Verification items for the finished model (mm, model axes). A direction names the side the tool comes from. Coordinates: 2 decimals unless noted, no trailing zeros. Write each loop counter-clockwise with the first axis right and the second up, starting at its lowest first coordinate (ties: lowest second). Pieces come first, ordered by that corner, then holes. Notation, with made-up numbers: M 80,78 L 89,78 A24 ccw 89,93 Z; hole C 17,41 d10. An arc over 180 degrees is marked long. Answer in a Markdown table with one row per item.
Autodesk Inventor part; units mm, degrees
ref_plane "YZ Plane" through (0, 0, 0) normal (1, 0, 0) x (0, 1, 0)
ref_plane "XZ Plane" through (0, 0, 0) normal (0, 1, 0) x (-1, 0, 0)
ref_plane "XY Plane" through (0, 0, 0) normal (0, 0, 1) x (1, 0, 0)
sketch "Sketch1" plane through (0, 0, 0) normal (0, 0, 1) x (1, 0, 0)
  line L0 (0, 0) -> (6.223, 0)
  line L1 (0, 0) -> (6.223, 0) construction
  line L2 (6.223, 0) -> (6.223, 38.1)
  line L3 (0, 0) -> (0.762, 0)
  line L4 (0.762, 0) -> (0.762, 8.255)
  line L5 (0.762, 8.255) -> (6.223, 28.635729)
  line L6 (6.223, 28.635729) -> (6.223, 38.1)
  line L7 (0, 0) -> (12.7, 0)
  line L8 (0, -8.9154) -> (0, 53.4924)
  line L9 (6.223, 38.1) -> (12.20332, 44.08032)
  line L10 (6.223, 38.1) -> (14.68045, 38.1) construction
  line L11 (12.20332, 44.08032) -> (12.7, 0)
  line L12 (12.7, 0) -> (12.7, 44.577)
  line L13 (12.7, 44.577) -> (6.223, 38.1)
  line L14 (6.223, 38.1) -> (0, 38.1)
  line L15 (0, 8.255) -> (0.762, 8.255)
  line L16 (0, 8.255) -> (0, 38.1)
  line L17 (6.223, 28.635729) -> (0, 28.635729)
  line L18 (0, 28.635729) -> (8.60425, 28.635729)
  line L19 (8.60425, 28.635729) -> (0.762, 8.255)
  line L20 (8.60425, 28.635729) -> (8.60425, 40.48125)
  dimension "d0" = 6.223
  dimension "d1" = 0
  dimension "d2" = 38.1
  dimension "d3" = 90
  dimension "d4" = 0.762
  dimension "d5" = 8.255
  dimension "d6" = 165
  dimension "d7" = 12.7
  dimension "d18" = 45
  dimension "d58" = 8.60425
sketch "Sketch1 outline for Revolution1" plane through (0, 0, 0) normal (0, 0, 1) x (1, 0, 0)
  line L0 (8.60425, 40.48125) -> (8.60425, 28.635729)
  line L1 (8.60425, 28.635729) -> (0.762, 8.255)
  line L2 (0.762, 8.255) -> (0.762, 0)
  line L3 (0.762, 0) -> (12.7, 0)
  line L4 (12.7, 0) -> (12.7, 44.577)
  line L5 (12.7, 44.577) -> (8.60425, 40.48125)
revolve "Revolution1" add sketch "Sketch1 outline for Revolution1" angle 360 about axis through (0, -10, 0) along (0, 1, 0)
sketch "Sketch3" plane through (0, 0, 0) normal (0, -1, 0) x (1, 0, 0)
  point P0 (0, 0)
  point P1 (0, 0)
hole "Hole2" at (0, 0, 0) direction (0, 1, 0) diameter 5.3594 depth 6.35
sketch "Sketch4" plane through (0, 0, 0) normal (1, 0, 0) x (0, 1, 0)
  line L0 (0, 12.7) -> (0, -12.7)
  line L1 (0, 12.7) -> (0, 7.9248)
  line L2 (0, 7.9248) -> (12.7, 7.9248)
  line L3 (0, -12.7) -> (0, -7.9248)
  line L4 (0, -7.9248) -> (12.7, -7.9248)
  point P0 (0, 0)
  dimension "d28" = 4.7752
  dimension "d29" = 12.7
  dimension "d30" = 4.7752
  dimension "d31" = 12.7
  dimension "d32" = 90
hole "Hole3" at (0, 12.7, 7.9248) at (0, 12.7, -7.9248) direction (-1, 0, 0) diameter 4.4958 end through all
mirror "Mirror1" about plane through (0, 0, 0) normal (1, 0, 0) of "Hole3"
equation "\"d47\" = 55deg"
equation "\"Sketch5_Pitch\" = 0.90714"
properties part number "catch vertical seal-tighttol-thread"
1) Thickness scan on L1, parallel to Z at x = 0, y = 7.8; L2, parallel to X at y = 3.5, z = 0; L3, parallel to Z at x = -4.25, y = 12.5. Record the ranges inside material, lowest first. Write a range as [from, to].
Response values:
| item | result |
|---|---|
| L1 | z = [-12.7, -0.76], [0.76, 12.7] |
| L2 | x = [-12.7, -2.68], [2.68, 12.7] |
| L3 | z = [-11.97, -10.16], [-5.69, 5.69], [10.16, 11.97] |
2) Sectioned sample at D-D (y = 33). Record the cut outline in (x, z), then the cut area to 3 significant figures.
Response values:
| item | result |
|---|---|
| outline | C 0,0 d25.4; hole C 0,0 d17.21 |
| area | 274 mm² |
3) Release check for a two-part mould opening along X. For faces 4 (the face through (12.114, 22.601, -3.815)), 5 (the face through (-1.92, 40.74, 8.65)), 6 (the face through (0.16, 12.8, -5.68)) record: +X half, -X half, draft (parallel to the pull), parting line (faces both ways), or undercut.
Response values:
| item | result |
|---|---|
| face 4 | parting line |
| face 5 | undercut |
| face 6 | draft |
4) Depth check by flat-ended pin: pin 1 (6 mm diameter, centred on y = 12.7, z = 7.92, fed in from -X); pin 2 (12 mm diameter, centred on x = 3, z = 8.5, fed in from -Y); pin 3 (1 mm diameter, centred on y = 8, z = 1, fed in from +X); pin 4 (1 mm diameter, centred on x = 1, y = 6, fed in from +Z). Enter the tip coordinate at first touch or a pass-through.
Response values:
| item | result |
|---|---|
| pin 1 | stops at x = -11.71 |
| pin 2 | stops at y = 0 |
| pin 3 | stops at x = 12.69 |
| pin 4 | stops at z = 12.69 |
5) Tool access check on faces 1 (the face through (0, 0, -3)), 2 (the face through (-1.87, 34.48, -8.4)), 3 (the face through (-0.118, 3.219, 2.677)). Record the directions out of +Z, -Z, +X, -X, +Y, -Y that give a thin tool (end or side, any length) a straight path to the whole face; none if there is none.
Response values:
| item | result |
|---|---|
| face 1 | +Z, -Z, +X, -X, -Y |
| face 2 | +Y |
| face 3 | -Y |
6) Sectioned sample at C-C (y = 12.7). Record the cut outline in (x, z), then the cut area to 3 significant figures.
Response values:
| item | result |
|---|---|
| outline | M -11.36,-5.68 L 11.36,-5.68 A12.7 ccw 11.36,5.68 L -11.36,5.68 A12.7 ccw Z; M -7.6,-10.17 A12.7 ccw 7.6,-10.17 Z; M -7.6,10.17 L 7.6,10.17 A12.7 ccw Z; hole C 0,0 d4.94 |
| area | 312 mm² |
7) Sectioned sample at A-A (x = 0). Record the cut outline in (y, z) (3 decimals), then the cut area to 3 significant figures.
Response values:
| item | result |
|---|---|
| outline | M 0,-12.7 L 44.577,-12.7 L 40.481,-8.604 L 28.636,-8.604 L 8.255,-0.762 L 6.35,-0.762 L 6.35,-2.68 L 0,-2.68 Z; M 0,2.68 L 6.35,2.68 L 6.35,0.762 L 8.255,0.762 L 28.636,8.604 L 40.481,8.604 L 44.577,12.7 L 0,12.7 Z; hole C 12.7,-7.925 d4.496; hole C 12.7,7.925 d4.496 |
| area | 582 mm² |
8) Sectioned sample at B-B (z = 0). Record the cut outline in (x, y) (3 decimals), then the cut area to 3 significant figures.
Response values:
| item | result |
|---|---|
| outline | M -12.7,0 L -2.68,0 L -2.68,6.35 L -0.762,6.35 L -0.762,8.255 L -8.604,28.636 L -8.604,40.481 L -12.7,44.577 Z; M 0.762,6.35 L 2.68,6.35 L 2.68,0 L 12.7,0 L 12.7,44.577 L 8.604,40.481 L 8.604,28.636 L 0.762,8.255 Z |
| area | 613 mm² |
